CAD build for the part. Positions are in the model's coordinates, mm. A direction names the side the tool comes from. Round coordinates to 2 decimals unless told otherwise and drop trailing zeros. Answer as CSV lines item,"result". Start each with the question number.
```python
from build123d import *

# Parameters (mm, degrees)
BOSS_EXTRUDE1_DEPTH     = 4
SKETCH2_R               = 0.62500002
CUT_EXTRUDE1_DEPTH      = 2.44
CUT_EXTRUDE3_DEPTH      = 54.906897466
CUT_EXTRUDE3_DEPTH_BACK = 54.906897466
SKETCH3_R               = 0.62500002
SKETCH3_R_2             = 2.819999948
SKETCH3_R_3             = 2.899999788


with BuildPart() as part:
    # Sketch1 → Boss-Extrude1 (new body)
    with BuildSketch(Plane(origin=(0, 0, 0), x_dir=(1, 0, 0), z_dir=(0, 1, 0))):
        with BuildLine():
            Line((-29.999999944, 20), (29.999999944, 20))
            ThreePointArc((29.999999944, 20), (49.999999944, 0), (29.999999944, -20))
            Line((29.999999944, -20), (-29.999999944, -20))
            ThreePointArc((-29.999999944, -20), (-49.999999944, 0), (-29.999999944, 20))
        make_face()
    extrude(amount=BOSS_EXTRUDE1_DEPTH)

    # Sketch2 → Cut-Extrude1 (cut)
    # profile 1 of 2: a face of its own
    with BuildSketch(Plane(origin=(0, 4, 0), x_dir=(1, 0, 0), z_dir=(0, 1, 0))):
        with BuildLine():
            ThreePointArc((23.401904925, 3.184398134), (25.657534853, 4.342465091), (26.81560181, 6.598095019))
            Line((26.81560181, 6.598095019), (28.026588273, 13.950499547))
            ThreePointArc((28.026588273, 13.950499547), (29.999999943, 15.239999998), (31.973411615, 13.950499548))
            Line((31.973411615, 13.950499548), (33.184398078, 6.598095019))
            ThreePointArc((33.184398078, 6.598095019), (34.342465035, 4.342465091), (36.598094963, 3.184398134))
            Line((36.598094963, 3.184398134), (43.950499491, 1.973411671))
            ThreePointArc((43.950499491, 1.973411671), (45.239999942, 1e-09), (43.950499492, -1.973411671))
            Line((43.950499492, -1.973411671), (36.598094963, -3.184398134))
            ThreePointArc((36.598094963, -3.184398134), (34.342465035, -4.342465091), (33.184398078, -6.598095019))
            Line((33.184398078, -6.598095019), (31.973411615, -13.950499547))
            ThreePointArc((31.973411615, -13.950499547), (29.999999945, -15.239999998), (28.026588273, -13.950499548))
            Line((28.026588273, -13.950499548), (26.81560181, -6.598095019))
            ThreePointArc((26.81560181, -6.598095019), (25.657534853, -4.342465091), (23.401904925, -3.184398134))
            Line((23.401904925, -3.184398134), (16.049500397, -1.973411671))
            ThreePointArc((16.049500397, -1.973411671), (14.759999946, -1e-09), (16.049500396, 1.973411671))
            Line((16.049500396, 1.973411671), (23.401904925, 3.184398134))
        make_face()
        with Locations(Location((16.499533422, 0, 0), (0, 0, 270))):
            Circle(SKETCH2_R, mode=Mode.SUBTRACT)
        with Locations(Location((22.499533614, 0, 0), (0, 0, 270))):
            Circle(SKETCH2_R, mode=Mode.SUBTRACT)
        with Locations(Location((19.499533518, 0, 0), (0, 0, 270))):
            Circle(SKETCH2_R, mode=Mode.SUBTRACT)
        with Locations(Location((43.500466466, 0, 0), (0, 0, 270))):
            Circle(SKETCH2_R, mode=Mode.SUBTRACT)
        with Locations(Location((37.500466274, 0, 0), (0, 0, 270))):
            Circle(SKETCH2_R, mode=Mode.SUBTRACT)
        with Locations(Location((40.50046637, 0, 0), (0, 0, 270))):
            Circle(SKETCH2_R, mode=Mode.SUBTRACT)
        with Locations(Location((29.999999944, 7.50046633, 0), (0, 0, 270))):
            Circle(SKETCH2_R, mode=Mode.SUBTRACT)
        with Locations(Location((29.999999944, 10.500466426, 0), (0, 0, 270))):
            Circle(SKETCH2_R, mode=Mode.SUBTRACT)
        with Locations(Location((29.999999944, 13.500466522, 0), (0, 0, 270))):
            Circle(SKETCH2_R, mode=Mode.SUBTRACT)
        with Locations(Location((29.999999944, -13.500466522, 0), (0, 0, 270))):
            Circle(SKETCH2_R, mode=Mode.SUBTRACT)
        with Locations(Location((29.999999944, -10.500466426, 0), (0, 0, 270))):
            Circle(SKETCH2_R, mode=Mode.SUBTRACT)
        with Locations(Location((29.999999944, -7.50046633, 0), (0, 0, 270))):
            Circle(SKETCH2_R, mode=Mode.SUBTRACT)
    # profile 2 of 2: a face of its own
    with BuildSketch(Plane(origin=(0, 4, 0), x_dir=(1, 0, 0), z_dir=(0, 1, 0))):
        with BuildLine():
            Line((-26.859652917, 6.619867525), (-28.07063938, 13.972272054))
            ThreePointArc((-28.07063938, 13.972272054), (-30.044051051, 15.261772506), (-32.017462722, 13.972272054))
            Line((-32.017462722, 13.972272054), (-33.228449185, 6.619867525))
            ThreePointArc((-33.228449185, 6.619867525), (-33.569143262, 6.127411318), (-34.165969886, 6.078589696))
            Line((-34.165969886, 6.078589696), (-41.138832219, 8.70604692))
            ThreePointArc((-41.138832219, 8.70604692), (-43.242278204, 7.641772507), (-43.112243889, 5.287997642))
            Line((-43.112243889, 5.287997642), (-37.35036802, 0.563050336))
            ThreePointArc((-37.35036802, 0.563050336), (-37.094235473, 0.021772507), (-37.35036802, -0.519505322))
            Line((-37.35036802, -0.519505322), (-43.112243889, -5.244452627))
            ThreePointArc((-43.112243889, -5.244452627), (-43.242278204, -7.598227492), (-41.138832218, -8.662501905))
            Line((-41.138832218, -8.662501905), (-34.165969886, -6.035044681))
            ThreePointArc((-34.165969886, -6.035044681), (-33.569143262, -6.083866304), (-33.228449185, -6.57632251))
            Line((-33.228449185, -6.57632251), (-32.017462722, -13.928727039))
            ThreePointArc((-32.017462722, -13.928727039), (-30.044051051, -15.218227491), (-28.07063938, -13.928727039))
            Line((-28.07063938, -13.928727039), (-26.859652917, -6.576322511))
            ThreePointArc((-26.859652917, -6.576322511), (-26.51895884, -6.083866304), (-25.922132216, -6.035044681))
            Line((-25.922132216, -6.035044681), (-18.949269883, -8.662501905))
            ThreePointArc((-18.949269883, -8.662501905), (-16.845823898, -7.598227492), (-16.975858213, -5.244452627))
            Line((-16.975858213, -5.244452627), (-22.737734082, -0.519505322))
            ThreePointArc((-22.737734082, -0.519505322), (-22.993866629, 0.021772507), (-22.737734082, 0.563050336))
            Line((-22.737734082, 0.563050336), (-16.975858213, 5.287997642))
            ThreePointArc((-16.975858213, 5.287997642), (-16.845823898, 7.641772507), (-18.949269884, 8.70604692))
            Line((-18.949269884, 8.70604692), (-25.922132216, 6.078589696))
            ThreePointArc((-25.922132216, 6.078589696), (-26.51895884, 6.127411318), (-26.859652917, 6.619867525))
        make_face()
    extrude(amount=-CUT_EXTRUDE1_DEPTH, mode=Mode.SUBTRACT)

    # Sketch3 → Cut-Extrude3 (cut, two sides: drawn at the far end of the back side and taken through both)
    with BuildSketch(Plane(origin=(0, 1.56, 0), x_dir=(1, 0, 0), z_dir=(0, 1, 0)).offset(-CUT_EXTRUDE3_DEPTH_BACK)):
        with Locations(Location((-30.044051051, 13.522239028, 0), (0, 0, 270))):
            Circle(SKETCH3_R)
        with Locations(Location((-30.044051051, 10.522238932, 0), (0, 0, 270))):
            Circle(SKETCH3_R)
        with Locations(Location((-30.044051051, 7.522238836, 0), (0, 0, 270))):
            Circle(SKETCH3_R)
        with Locations(Location((-23.548456669, 3.772005671, 0), (0, 0, 270))):
            Circle(SKETCH3_R)
        with Locations(Location((-20.950380374, 5.272005719, 0), (0, 0, 270))):
            Circle(SKETCH3_R)
        with Locations(Location((-18.35230408, 6.772005767, 0), (0, 0, 270))):
            Circle(SKETCH3_R)
        with Locations(Location((-23.548456669, -3.728460659, 0), (0, 0, 270))):
            Circle(SKETCH3_R)
        with Locations(Location((-20.950380374, -5.228460707, 0), (0, 0, 270))):
            Circle(SKETCH3_R)
        with Locations(Location((-18.35230408, -6.728460755, 0), (0, 0, 270))):
            Circle(SKETCH3_R)
        with Locations(Location((-30.044051051, -7.478693824, 0), (0, 0, 270))):
            Circle(SKETCH3_R)
        with Locations(Location((-30.044051051, -10.47869392, 0), (0, 0, 270))):
            Circle(SKETCH3_R)
        with Locations(Location((-30.044051051, -13.478694016, 0), (0, 0, 270))):
            Circle(SKETCH3_R)
        with Locations(Location((-36.539645433, -3.728460659, 0), (0, 0, 270))):
            Circle(SKETCH3_R)
        with Locations(Location((-39.137721727, -5.228460707, 0), (0, 0, 270))):
            Circle(SKETCH3_R)
        with Locations(Location((-41.735798022, -6.728460755, 0), (0, 0, 270))):
            Circle(SKETCH3_R)
        with Locations(Location((-36.539645433, 3.772005671, 0), (0, 0, 270))):
            Circle(SKETCH3_R)
        with Locations(Location((-39.137721727, 5.272005719, 0), (0, 0, 270))):
            Circle(SKETCH3_R)
        with Locations(Location((-41.735798022, 6.772005767, 0), (0, 0, 270))):
            Circle(SKETCH3_R)
        with Locations(Location((-30.044051051, 0.021772506, 0), (0, 0, 270))):
            Circle(SKETCH3_R_2)
        with Locations(Location((29.999999944, 0, 0), (0, 0, 270))):
            Circle(SKETCH3_R_3)
        with Locations(Location((29.999999944, 7.50046633, 0), (0, 0, 270))):
            Circle(SKETCH3_R)
        with Locations(Location((29.999999944, 10.500466426, 0), (0, 0, 270))):
            Circle(SKETCH3_R)
        with Locations(Location((29.999999944, 13.500466522, 0), (0, 0, 270))):
            Circle(SKETCH3_R)
        with Locations(Location((16.499533422, 0, 0), (0, 0, 270))):
            Circle(SKETCH3_R)
        with Locations(Location((19.499533518, 0, 0), (0, 0, 270))):
            Circle(SKETCH3_R)
        with Locations(Location((22.499533614, 0, 0), (0, 0, 270))):
            Circle(SKETCH3_R)
        with Locations(Location((29.999999944, -13.500466522, 0), (0, 0, 270))):
            Circle(SKETCH3_R)
        with Locations(Location((29.999999944, -10.500466426, 0), (0, 0, 270))):
            Circle(SKETCH3_R)
        with Locations(Location((29.999999944, -7.50046633, 0), (0, 0, 270))):
            Circle(SKETCH3_R)
        with Locations(Location((43.500466466, 0, 0), (0, 0, 270))):
            Circle(SKETCH3_R)
        with Locations(Location((40.50046637, 0, 0), (0, 0, 270))):
            Circle(SKETCH3_R)
        with Locations(Location((37.500466274, 0, 0), (0, 0, 270))):
            Circle(SKETCH3_R)
    extrude(amount=CUT_EXTRUDE3_DEPTH + CUT_EXTRUDE3_DEPTH_BACK, mode=Mode.SUBTRACT)


solid = part.part
```
Q1. Probe line 1 along X through (y, z) = (2.45, -15); line 2 along Z through (x, y) = (-42.5, 1.95); line 3 along Z through (x, y) = (-19.5, 1.65). List the from-to ranges inside material, lowest first. Write a range as from..to.
Q2. Tool access for faces 1 (the cylindrical face through (-32.797, 0.769, -0.633)), 2 (the flat face through (40.223, 2.797, -2.587)): list every direction of +Z, -Z, +X, -X, +Y, -Y with a clear straight run to the whole face (end or side of a thin tool).
Q3. Drop flat-ended pins along their axis: P1, Ø0.8, axis at x = -23.55, z = -3.77, coming from the +Y side; P2, Ø2, axis at x = 19.5, z = 0, coming from the +Y side; P3, Ø2, axis at y = 3, z = -0.5, coming from the +X side. Give the stop position or say it passes through.
Q4. Mould opens along Z. For faces 3 (the cylindrical face through (45.24, 2.8, -0.03)), 4 (the flat face through (1, 4, 0)), 5 (the flat face through (0, 2, -20)), 6 (the flat face through (-32.614, 2.797, -10.348)) say: +Z half, -Z half, draft (parallel to the pull), parting line (faces both ways), or undercut.
Q5. Band-saw the part on A-A, the plane y = 3.15. Count the separate pieces of the cut face and the enclosed holes in it, then the cut area to 3 significant figures.
Answer:
1,line 1,"x = -43.23..-31.07, -29.01..29.01, 30.99..43.23"
1,line 2,"z = -15.61..-8.4, -4.79..4.74, 8.36..15.61"
1,line 3,"z = -20..-8.5, -3.22..3.17, 8.45..20"
2,face 1,"+Y, -Y"
2,face 2,"+Y"
3,P1,"passes through"
3,P2,"stops at y = 1.56"
3,P3,"stops at x = 50"
4,face 3,"undercut"
4,face 4,"draft"
4,face 5,"-Z half"
4,face 6,"undercut"
5,separate pieces,"1"
5,enclosed holes,"2"
5,area,"2,950 mm^2"
